```python
from build123d import *
from OCP.BRepFilletAPI import BRepFilletAPI_MakeChamfer

# Parameters (mm, degrees)
BOSS_EXTRUDE1_DEPTH = 2.54
CHAMFER2_SIZE       = 1.143
CHAMFER2_SIZE2      = 4.265734073


with BuildPart() as part:
    # Sketch1 → Boss-Extrude1 (new body)
    with BuildSketch(Plane.XY):
        Polygon((0, 0), (355.6, 0), (304.8, 88.9), (254, 88.9), align=None)
    extrude(amount=BOSS_EXTRUDE1_DEPTH)

    # Chamfer2: one chamfer whose edges measure the first distance from different faces: ONE call of the kernel's chamfer builder (chamfer() names one face for all edges)
    chamfer2_edges_1 = [part.edges().sort_by_distance(p)[0] for p in [
        (330.2, 44.45, 2.54),
        (330.2, 44.45, 0),
    ]]
    chamfer2_side_1 = [part.faces().sort_by_distance(p)[0] for p in [
        (330.2, 44.45, 1.27),
    ]]
    chamfer2_edges_2 = [part.edges().sort_by_distance(p)[0] for p in [
        (127, 44.45, 2.54),
        (127, 44.45, 0),
    ]]
    chamfer2_side_2 = [part.faces().sort_by_distance(p)[0] for p in [
        (127, 44.45, 1.27),
    ]]
    chamfer2 = BRepFilletAPI_MakeChamfer(part.part.solid().wrapped)
    for e in chamfer2_edges_1:
        chamfer2.Add(CHAMFER2_SIZE, CHAMFER2_SIZE2, e.wrapped, chamfer2_side_1[0].wrapped)  # the first distance lies on this face
    for e in chamfer2_edges_2:
        chamfer2.Add(CHAMFER2_SIZE, CHAMFER2_SIZE2, e.wrapped, chamfer2_side_2[0].wrapped)  # the first distance lies on this face
    add(Compound.cast(chamfer2.Shape()), mode=Mode.REPLACE)


solid = part.part
```
Can you work these out from the model? Positions are in its coordinate system, mm. Coordinates: 2 decimals unless noted, no trailing zeros. Loops run counter-clockwise (first coordinate to the right, second up) from the corner with the lowest first, then second, coordinate; pieces in that order, holes last. Notation, with made-up numbers: (-6, 40.5) - (8, 40.5) arc R28 ccw to (8, 69.5) - close; hole circle Ø11 at (13, 18.5). An arc over 180 degrees is marked (long way). Use a Markdown table: item, result.
Item 1: I want a section at D-D on z = 0.55. Please give me the cut outline in (x, y).
Numbers:
| item | result |
|---|---|
| outline | (6.7, 0) - (353.05, 0) - (302.25, 88.9) - (260.7, 88.9) - close |
Item 2: I want a section at B-B on x = 187.5. Please give me the cut outline in (y, z) (3 decimals).
Numbers:
| item | result |
|---|---|
| outline | (0, 0) - (61.106, 0) - (65.625, 1.143) - (65.625, 1.397) - (61.106, 2.54) - (0, 2.54) - close |
Item 3: I want a section at A-A on y = 65.5. Please give me the cut outline in (x, z).
Numbers:
| item | result |
|---|---|
| outline | (187.14, 1.14) - (200.06, 0) - (313.26, 0) - (318.17, 1.14) - (318.17, 1.4) - (313.26, 2.54) - (200.06, 2.54) - (187.14, 1.4) - close |
Item 4: I want a section at C-C on y = 9. Please give me the cut outline in (x, z).
Numbers:
| item | result |
|---|---|
| outline | (25.71, 1.14) - (38.63, 0) - (345.54, 0) - (350.46, 1.14) - (350.46, 1.4) - (345.54, 2.54) - (38.63, 2.54) - (25.71, 1.4) - close |
Item 5: If I drill on probe 1 along Z at (x, y) = (79.5, 26.5); probe 2 along Z at (x, y) = (40, 11.5), over which ranges is the centre line in solid material (lowest first)? Write a range as from..to.
Numbers:
| item | result |
|---|---|
| probe 1 | z = 0.81..1.73 |
| probe 2 | z = 0.51..2.03 |
